Geometry check sheet. Reference: the model listing, model coordinates, mm. A direction names the side the tool comes from. Coordinates: 2 decimals unless noted, no trailing zeros. Order: outer loops, then holes, each group sorted by start corner. A loop starts at its lowest first (then second) coordinate and runs counter-clockwise, first axis right, second up. Notation, with made-up numbers: M 71,-3 L 86,-3 A19 cw 86,1 Z; hole C -37.75,-2.5 d2. An arc over 180 degrees is marked long. Use CSV: the item, a comma, the result in double quotes. Start each with the question number.
```python
from build123d import *

# Parameters (mm, degrees)
SKICA2_R                = 2.35
SKICA2_W                = 11
SKICA2_H                = 3.499027085
SKICA2_W_2              = 3
SKICA2_H_2              = 13
SKICA2_W_3              = 3.2
SKICA2_H_3              = 10
SKICA2_W_4              = 3.215746781
P_IDAT_VYSUNUT_M1_DEPTH = 3


with BuildPart() as part:
    # Skica2 → Přidat vysunutím1 (new body)
    with BuildSketch(Plane.XY):
        with BuildLine():
            Line((-62.5, 7.5), (-61.3, 7.5))
            ThreePointArc((-61.3, 7.5), (-52.847781356, 11.3), (-44.395562713, 7.5))
            Line((-44.395562713, 7.5), (-44.395562713, 3))
            Line((-44.395562713, 3), (-41.953287334, 3))
            ThreePointArc((-41.953287334, 3), (-41.547781356, 0), (-41.953287334, -3))
            Line((-41.953287334, -3), (-44.395562713, -3))
            Line((-44.395562713, -3), (-44.395562713, -7.5))
            ThreePointArc((-44.395562713, -7.5), (-52.847781356, -11.3), (-61.3, -7.5))
            Line((-61.3, -7.5), (-62.5, -7.5))
            Line((-62.5, -7.5), (-62.5, -16.780342451))
            Line((-62.5, -16.780342451), (-62.5, -31.5))
            ThreePointArc((-62.5, -31.5), (-54.884776311, -49.884776311), (-36.5, -57.5))
            Line((-36.5, -57.5), (-32.5, -57.5))
            ThreePointArc((-32.5, -57.5), (-22.600505063, -53.399494937), (-18.5, -43.5))
            Line((-18.5, -43.5), (-18.5, -42.5))
            ThreePointArc((-18.5, -42.5), (-15.571067812, -35.428932188), (-8.5, -32.5))
            Line((-8.5, -32.5), (8.5, -32.5))
            ThreePointArc((8.5, -32.5), (15.571067812, -35.428932188), (18.5, -42.5))
            Line((18.5, -42.5), (18.5, -43.5))
            ThreePointArc((18.5, -43.5), (22.600505063, -53.399494937), (32.5, -57.5))
            Line((32.5, -57.5), (36.5, -57.5))
            ThreePointArc((36.5, -57.5), (54.884776311, -49.884776311), (62.5, -31.5))
            Line((62.5, -31.5), (62.5, -18.974988021))
            Line((62.5, -18.974988021), (62.5, -7.5))
            Line((62.5, -7.5), (61.3, -7.5))
            ThreePointArc((61.3, -7.5), (52.847781356, -11.3), (44.395562713, -7.5))
            Line((44.395562713, -7.5), (44.395562713, -3))
            Line((44.395562713, -3), (41.953287334, -3))
            ThreePointArc((41.953287334, -3), (41.547781356, 0), (41.953287334, 3))
            Line((41.953287334, 3), (44.395562713, 3))
            Line((44.395562713, 3), (44.395562713, 7.5))
            ThreePointArc((44.395562713, 7.5), (52.847781356, 11.3), (61.3, 7.5))
            Line((61.3, 7.5), (62.5, 7.5))
            Line((62.5, 7.5), (62.5, 17.5))
            ThreePointArc((62.5, 17.5), (58.106601718, 28.106601718), (47.5, 32.5))
            Line((47.5, 32.5), (43, 32.5))
            ThreePointArc((43, 32.5), (41.939339828, 32.939339828), (41.5, 34))
            Line((41.5, 34), (41.5, 34.5))
            ThreePointArc((41.5, 34.5), (40.328427125, 37.328427125), (37.5, 38.5))
            Line((37.5, 38.5), (-37.5, 38.5))
            ThreePointArc((-37.5, 38.5), (-40.328427125, 37.328427125), (-41.5, 34.5))
            Line((-41.5, 34.5), (-41.5, 34))
            ThreePointArc((-41.5, 34), (-41.939339828, 32.939339828), (-43, 32.5))
            Line((-43, 32.5), (-47.5, 32.5))
            ThreePointArc((-47.5, 32.5), (-58.106601718, 28.106601718), (-62.5, 17.5))
            Line((-62.5, 17.5), (-62.5, 7.5))
        make_face()
        with Locations((-36, 18.55)):
            Circle(SKICA2_R, mode=Mode.SUBTRACT)
        with Locations((-36, -29.45)):
            Circle(SKICA2_R, mode=Mode.SUBTRACT)
        with Locations((36, -29.45)):
            Circle(SKICA2_R, mode=Mode.SUBTRACT)
        with Locations((36, 18.55)):
            Circle(SKICA2_R, mode=Mode.SUBTRACT)
        with Locations((-38.447781356, -46.193013209)):
            Rectangle(SKICA2_W, SKICA2_H, mode=Mode.SUBTRACT)
        with Locations((-38.447781356, -38.693986123)):
            Rectangle(SKICA2_W, SKICA2_H, mode=Mode.SUBTRACT)
        with Locations((-43.047781356, -20.7)):
            Rectangle(SKICA2_W_2, SKICA2_H_2, mode=Mode.SUBTRACT)
        with Locations((-43.047781356, 20.7)):
            Rectangle(SKICA2_W_2, SKICA2_H_2, mode=Mode.SUBTRACT)
        with Locations((43.047781356, -20.7)):
            Rectangle(SKICA2_W_2, SKICA2_H_2, mode=Mode.SUBTRACT)
        with Locations((43.047781356, 20.7)):
            Rectangle(SKICA2_W_2, SKICA2_H_2, mode=Mode.SUBTRACT)
        with Locations((-36.947781356, 30.5)):
            Rectangle(SKICA2_W_3, SKICA2_H_3, mode=Mode.SUBTRACT)
        with Locations((36.947781356, 30.5)):
            Rectangle(SKICA2_W_3, SKICA2_H_3, mode=Mode.SUBTRACT)
        with Locations((30.747781356, 30.5)):
            Rectangle(SKICA2_W_3, SKICA2_H_3, mode=Mode.SUBTRACT)
        with Locations((24.547781356, 30)):
            Rectangle(SKICA2_W_3, SKICA2_H_2, mode=Mode.SUBTRACT)
        with Locations((35.447781356, -38.693986123)):
            Rectangle(SKICA2_W, SKICA2_H, mode=Mode.SUBTRACT)
        with Locations((-30.739907966, 30.5)):
            Rectangle(SKICA2_W_4, SKICA2_H_3, mode=Mode.SUBTRACT)
        with Locations((-24.532034575, 30.5)):
            Rectangle(SKICA2_W_3, SKICA2_H_3, mode=Mode.SUBTRACT)
        with Locations((-18.332034575, 30.5)):
            Rectangle(SKICA2_W_3, SKICA2_H_3, mode=Mode.SUBTRACT)
        with Locations((18.347781356, 30.5)):
            Rectangle(SKICA2_W_3, SKICA2_H_3, mode=Mode.SUBTRACT)
        with Locations((35.447781356, -46.193013209)):
            Rectangle(SKICA2_W, SKICA2_H, mode=Mode.SUBTRACT)
    extrude(amount=P_IDAT_VYSUNUT_M1_DEPTH)


solid = part.part
```
1) Section check A-A on y = -29.45. Record the boundary of the cut face in (x, z).
2) Set-up check for faces 4 (the face through (-32.948, -39, 1)), 5 (the face through (54.68, -50.09, 1.48)): record each of +Z, -Z, +X, -X, +Y, -Y from which the full face is reachable in a straight line by a thin tool's end or side.
3) Material ranges on line 1 along X through (y, z) = (-19.5, 1.95); line 2 along Y through (x, z) = (36, 2); line 3 along X through (y, z) = (22, 1.7), recorded low to high.
4) Gauge pin test, flat ends, axial feed: P1, Ø1, axis at x = 40, y = -47, coming from the +Z side; P2, Ø1.5, axis at y = -3.5, z = 2.5, coming from the -X side; P3, Ø0.9, axis at y = -39.5, z = 1.5, coming from the -X side; P4, Ø0.9, axis at x = -24, z = 1, coming from the -Y side. Record the tip position at first contact, or that the pin passes through.
5) Section check C-C on x = 0. Record the boundary of the cut face in (y, z).
6) Section check B-B on y = 29.5. State how many separate pieces and enclosed holes the cut face has, then the cut area to 3 significant figures.
7) Draft check along X on faces 1 (the face through (44.396, 5, 1)), 2 (the face through (-18, 35.5, 1)), 3 (the face through (-43, 3, 1)). Enter one of: +X half, -X half, draft (parallel to the pull), parting line (faces both ways), or undercut.
Results are:
1,outline,"M -62.5,0 L -38.35,0 L -38.35,3 L -62.5,3 Z; M -33.65,0 L 33.65,0 L 33.65,3 L -33.65,3 Z; M 38.35,0 L 62.5,0 L 62.5,3 L 38.35,3 Z"
2,face 4,"+Z, -Z"
2,face 5,"+Z, -Z, +X, -Y"
3,line 1,"x = -62.5 to -44.55, -41.55 to 41.55, 44.55 to 62.5"
3,line 2,"y = -57.5 to -47.94, -44.44 to -40.44, -36.94 to -31.8, -27.1 to 16.2, 20.9 to 25.5, 35.5 to 38.5"
3,line 3,"x = -61.81 to -44.55, -41.55 to 41.55, 44.55 to 61.81"
4,P1,"passes through"
4,P2,"stops at x = -44.4"
4,P3,"stops at x = -61.38"
4,P4,"stops at y = -54.95"
5,outline,"M -32.5,0 L 38.5,0 L 38.5,3 L -32.5,3 Z"
6,separate pieces,"9"
6,enclosed holes,"0"
6,area,"262 mm²"
7,face 1,"+X half"
7,face 2,"undercut"
7,face 3,"draft"
